Design review of the part built by this model. Coordinates are the model's own, in mm. A direction names the side the tool comes from. Coordinates: 2 decimals unless noted, no trailing zeros. Loops run counter-clockwise (first coordinate to the right, second up) from the corner with the lowest first, then second, coordinate; pieces in that order, holes last. Notation, with made-up numbers: (44, 38) -> (92, 38) arc R14 ccw to (92, 62) -> close; hole circle Ø4 at (62, 7). An arc over 180 degrees is marked (long way). Use a Markdown table: item, result. Add a question column.
Q1. Take a section at B-B on z = 0. Count the separate pieces of the cut face and the enclosed holes in it, plus the area to 3 significant figures.
Q2. Take a section at A-A on x = 19.5. Write out the cut boundary in (y, z), plus the area to 3 significant figures.
Q3. Clearance check with flat-ended pins moving along their axes: pin 1 Ø0.9 at (x, y) = (46, -13.5) entering from -Z; pin 2 Ø2 at (x, z) = (51, 67.5) entering from +Y; pin 3 Ø8 at (x, z) = (8, -84) entering from -Y; pin 4 Ø21.5 at (y, z) = (-62.5, 0) entering from +X. State where each tip first meets the part, or that it passes through.
Q4. For faces 5 (the face through (26.154, 20, 20)), 6 (the face through (16.87, 65.64, -85.61)), 7 (the face through (62.316, -7.509, 23.846)), list the 3-axis set-ups (+Z, -Z, +X, -X, +Y, -Y) from which the entire face can be reached by the end or side of a thin tool; tool diameter is ignored.
Q5. For probe 1 along X at (y, z) = (-53, -33.5); probe 2 along Z at (x, y) = (60, -83); probe 3 along Y at (x, z) = (39.25, -62.5), list the stretches that pass through material, from the lowest coordinate up.
Q6. Draft analysis for pull direction X (two halves, no side actions). For faces 1 (the face through (57.347, 95.926, 49.894)), 2 (the face through (0, -84, -56)), 3 (the face through (74.309, -84, 56)), 4 (the face through (11.99, -30.04, 95.38)), state which applies: pulls with the +X half, pulls with the -X half, needs draft (parallel to the pull), parting line crosses it, or undercut.
from build123d import *

# Parameters (mm, degrees)
SKETCH5_R          = 18
CUT_EXTRUDE1_DEPTH = 184.21802731
CUT_EXTRUDE2_DEPTH = 192.759733972


with BuildPart() as part:
    # Sketch1 → Revolve1 (revolve)
    with BuildSketch(Plane(origin=(0, 0, 0), x_dir=(1, 0, 0), z_dir=(0, 1, 0)), mode=Mode.PRIVATE) as revolve1_sk:
        with BuildLine():
            Line((0, 125), (0, 100))
            Line((0, 100), (23.65439265, 100))
            ThreePointArc((23.65439265, 100), (25.422159603, 99.267766953), (26.15439265, 97.5))
            Line((26.15439265, 97.5), (26.15439265, 27.5))
            ThreePointArc((26.15439265, 27.5), (25.422159603, 25.732233047), (23.65439265, 25))
            Line((23.65439265, 25), (2.5, 25))
            Line((2.5, 25), (0, 25))
            Line((0, 25), (0, 22.5))
            Line((0, 22.5), (0, 12.5))
            Line((0, 12.5), (74.308785301, 12.5))
            Line((74.308785301, 12.5), (74.308785301, 22.5))
            Line((74.308785301, 22.5), (74.308785301, 25))
            Line((74.308785301, 25), (71.808785301, 25))
            Line((71.808785301, 25), (50.65439265, 25))
            ThreePointArc((50.65439265, 25), (48.886625697, 25.732233047), (48.15439265, 27.5))
            Line((48.15439265, 27.5), (48.15439265, 97.5))
            ThreePointArc((48.15439265, 97.5), (48.886625697, 99.267766953), (50.65439265, 100))
            Line((50.65439265, 100), (74.308785301, 100))
            Line((74.308785301, 100), (74.308785301, 125))
            Line((74.308785301, 125), (69.308785301, 125))
            Line((69.308785301, 125), (62.757321084, 107))
            Line((62.757321084, 107), (57.757321084, 107))
            Line((57.757321084, 107), (51.205856867, 125))
            Line((51.205856867, 125), (46.205856867, 125))
            Line((46.205856867, 125), (39.65439265, 107))
            Line((39.65439265, 107), (34.65439265, 107))
            Line((34.65439265, 107), (28.102928434, 125))
            Line((28.102928434, 125), (23.102928434, 125))
            Line((23.102928434, 125), (16.551464217, 107))
            Line((16.551464217, 107), (11.551464217, 107))
            Line((11.551464217, 107), (5, 125))
            Line((5, 125), (0, 125))
        make_face()
    revolve(revolve1_sk.sketch.rotate(Axis((-67.943978181, 0, 0), (1, 0, 0)), 180), axis=Axis((-67.943978181, 0, 0), (1, 0, 0)))

    # Sketch5 → Cut-Extrude1 (cut, through all)
    with BuildSketch(Plane.ZY.offset(-26.15439265)):
        with Locations((0, 62.5)):
            Circle(SKETCH5_R)
        with Locations((62.5, 0)):
            Circle(SKETCH5_R)
        with Locations((0, -62.5)):
            Circle(SKETCH5_R)
        with Locations((-62.5, 0)):
            Circle(SKETCH5_R)
    extrude(amount=-CUT_EXTRUDE1_DEPTH, mode=Mode.SUBTRACT)

    # Sketch6 → Cut-Extrude2 (cut, through all)
    with BuildSketch(Plane.ZY):
        with BuildLine():
            Line((-3, -12.1346611), (-3, -15.1346611))
            Line((-3, -15.1346611), (3, -15.1346611))
            Line((3, -15.1346611), (3, -12.1346611))
            ThreePointArc((3, -12.1346611), (0, -12.5), (-3, -12.1346611))
        make_face()
    extrude(amount=-CUT_EXTRUDE2_DEPTH, mode=Mode.SUBTRACT)


solid = part.part
Answer list:
| question | item | result |
|---|---|---|
| 1 | separate pieces | 4 |
| 1 | enclosed holes | 0 |
| 1 | area | 5,860 mm² |
| 2 | outline | circle Ø230.2 at (0, 0); circle Ø50 at (0, 0); hole circle Ø200 at (0, 0); hole (-15.13, -3) -> (-12.13, -3) arc R12.5 ccw (long way) to (-12.13, 3) -> (-15.13, 3) -> close |
| 2 | area | 11,700 mm² |
| 3 | pin 1 | z = -124.31 |
| 3 | pin 2 | y = 105.84 |
| 3 | pin 3 | y = -94.9 |
| 3 | pin 4 | through |
| 4 | face 5 | -X |
| 4 | face 6 | none |
| 4 | face 7 | +X |
| 5 | probe 1 | 26.15 to 48.15 |
| 5 | probe 2 | -67.53 to -55.78, 55.78 to 67.53 |
| 5 | probe 3 | -86.85 to -18, 18 to 86.85 |
| 6 | face 1 | undercut |
| 6 | face 2 | pulls with the -X half |
| 6 | face 3 | pulls with the +X half |
| 6 | face 4 | needs draft |
